Can you work these out from the model? Positions are in its coordinate system, mm. A direction names the side the tool comes from. Round coordinates to 2 decimals unless told otherwise and drop trailing zeros. Order: outer loops, then holes, each group sorted by start corner. A loop starts at its lowest first (then second) coordinate and runs counter-clockwise, first axis right, second up. Notation, with made-up numbers: M 17.5,18 L 47.5,18 A19 ccw 47.5,35 Z; hole C 26.5,21 d6. An arc over 180 degrees is marked long. One line per question, with ' | ' between items.
```python
from build123d import *

# Parameters (mm, degrees)
SKETCH_2_R          = 5
CUT_EXTRUDE_1_DEPTH = 20
SKETCH_3_R          = 4
CUT_EXTRUDE_2_DEPTH = 81
SKETCH_4_R          = 4.5
CUT_EXTRUDE_3_DEPTH = 83.462112585
FILLET_1_R          = 5


with BuildPart() as part:
    # 草图1 → 旋转1 (revolve)
    with BuildSketch(Plane(origin=(0, 0, 0), x_dir=(1, 0, 0), z_dir=(0, 1, 0)), mode=Mode.PRIVATE) as revolve_1_sk:
        Polygon((0, 0), (40, 0), (40, -12), (15, -12), (15, -72), (0, -72), align=None)
    revolve(revolve_1_sk.sketch.rotate(Axis((0, 0, 0), (0, 0, 1)), 180), axis=Axis((0, 0, 0), (0, 0, 1)))

    # 草图2 → 切除-拉伸1 (cut)
    with BuildSketch(Plane.XY.offset(72)):
        Circle(SKETCH_2_R)
    extrude(amount=-CUT_EXTRUDE_1_DEPTH, mode=Mode.SUBTRACT)

    # 草图3 → 切除-拉伸2 (cut, symmetric)
    with BuildSketch(Plane(origin=(0, 0, 0), x_dir=(0, 0, -1), z_dir=(1, 0, 0))):
        with Locations((-40, 0)):
            Circle(SKETCH_3_R)
    extrude(amount=CUT_EXTRUDE_2_DEPTH, both=True, mode=Mode.SUBTRACT)

    # 草图4 → 切除-拉伸3 (cut, through all)
    with BuildSketch(Plane.XY.offset(12)):
        with Locations((21.213203, 21.213203)):
            Circle(SKETCH_4_R)
        with Locations((-21.213203, 21.213203)):
            Circle(SKETCH_4_R)
        with Locations((-21.213203, -21.213203)):
            Circle(SKETCH_4_R)
        with Locations((21.213203, -21.213203)):
            Circle(SKETCH_4_R)
    extrude(amount=-CUT_EXTRUDE_3_DEPTH, mode=Mode.SUBTRACT)

    # 圆角1
    fillet_1_edges = [part.edges().sort_by_distance(p)[0] for p in [
        (15, 0, 12),
    ]]
    fillet(fillet_1_edges, radius=FILLET_1_R)


solid = part.part
```
(1) Please list where these lines run through material, in increasing order: probe 1 along Y at (x, z) = (0, 67); probe 2 along Y at (x, z) = (0.5, 5.5); probe 3 along Z at (x, y) = (26.5, -18.5). Write a range as [from, to].
Final values:
probe 1: [-15, -5], [5, 15] | probe 2: [-40, 40] | probe 3: [0, 12]
(2) On a 3-axis mill with a long thin cutter (end or side, diameter ignored), from which of +Z, -Z, +X, -X, +Y, -Y can I reach the whole of each face in a straight line? I mean faces 4 (the flat face through (0, 0, 52)), 5 (the cylindrical face through (23.63, 25.01, 6.08)). Say none if no direction works.
Final values:
face 4: +Z | face 5: +Z, -Z
(3) If we section it at C-C on x = 24.5: Please give me the cut outline in (y, z), plus the area to 3 significant figures.
Final values:
outline: M -31.62,0 L -24.29,0 L -24.29,12 L -31.62,12 Z; M -18.14,0 L 18.14,0 L 18.14,12 L -18.14,12 Z; M 24.29,0 L 31.62,0 L 31.62,12 L 24.29,12 Z | area: 611 mm^2
(4) If we section it at A-A on y = 0: Please give me the cut outline in (x, z), plus the area to 3 significant figures.
Final values:
outline: M -40,0 L 40,0 L 40,12 L 20,12 A5 cw 15,17 L 15,36 L -15,36 L -15,17 A5 cw -20,12 L -40,12 Z; M -15,44 L 15,44 L 15,72 L 5,72 L 5,52 L -5,52 L -5,72 L -15,72 Z | area: 2,330 mm^2
(5) If we section it at D-D on z = 31.5: Please give me the cut outline in (x, y).
Final values:
outline: C 0,0 d30
(6) If we section it at B-B on x = 0: Please give me the cut outline in (y, z), plus the area to 3 significant figures.
Final values:
outline: M -40,0 L 40,0 L 40,12 L 20,12 A5 cw 15,17 L 15,72 L 5,72 L 5,52 L -5,52 L -5,72 L -15,72 L -15,17 A5 cw -20,12 L -40,12 Z; hole C 0,40 d8 | area: 2,520 mm^2
(7) Thinking about a two-plate mould opening in Z: for faces 1 (the flat face through (9.4, -18.3, 12)), 2 (the cylindrical face through (39.96, -1.76, 6.08)), 3 (the cylindrical face through (0.2, -2.4, 43.2)), which applies, released by +Z, released by -Z, zero draft, split by the parting line, or undercut?
Final values:
face 1: released by +Z | face 2: zero draft | face 3: undercut
(8) Will these pins go through, and if not, where does the flat tip stop? pin 1 Ø1.5 at (y, z) = (-16, 54.5) entering from -X; pin 2 Ø10 at (x, y) = (28.5, -2.5) entering from +Z; pin 3 Ø3 at (y, z) = (15, 8.5) entering from +X; pin 4 Ø5 at (x, z) = (-16, 29.5) entering from -Y.
Final values:
pin 1: through | pin 2: z = 12 | pin 3: x = 37.65 | pin 4: y = -6.54
